from build123d import *

# Parameters (mm, degrees)
F0_R     = 38.2508515855
F1_DEPTH = 17.526
F3_R     = 46.4966196034
F4_DEPTH = 12.7
F5_R     = 5.08
F6_W     = 8.4483027458
F6_H     = 6.8974085152
F8_DEPTH = 9.652
F7_W     = 9.7811389714
F7_H     = 6.7780073732
F9_DEPTH = 10.668


# Not quite as in the source:
# - a fillet or chamfer that OpenCascade refuses, or shapes differently, is made with other operations: its cross-section is extruded or revolved along the edge and cut away or added


with BuildPart() as f1:
    # F0 (on Top) → F1 (new body)
    with BuildSketch(Plane.XY):
        Circle(F0_R)
    extrude(amount=F1_DEPTH)

    # F2: fillet of radius 26.9812507731 on 1 edges, made by hand

    # F2_s1 → F2_t2 (revolve, cut)
    with BuildSketch(Plane.XZ):
        with BuildLine():
            ThreePointArc((38.2508515855, 0), (28.3570882092, 12.7157030349), (12.9805898912, 17.526))
            Line((12.9805898912, 17.526), (38.2508515855, 17.526))
            Line((38.2508515855, 17.526), (38.2508515855, 0))
        make_face()
    revolve(axis=Axis((0, 0, 17.526), (0, 0, 1)), mode=Mode.SUBTRACT)

    # F3 (on face) → F4 (join)
    with BuildSketch(Plane(origin=(0, 0, 0), x_dir=(1, 0, 0), z_dir=(0, 0, -1))):
        Circle(F3_R)
    extrude(amount=F4_DEPTH)

    # F5
    f5_edges = [f1.edges().sort_by_distance(p)[0] for p in [
        (-46.49662, 0, -12.7),
    ]]
    fillet(f5_edges, radius=F5_R)

    # F6 (on face) → F8 (join)
    with BuildSketch(Plane(origin=(0, 0, -12.7), x_dir=(1, 0, 0), z_dir=(0, 0, -1))):
        with Locations((-15.9282591194, 18.548514694)):
            Rectangle(F6_W, F6_H)
    extrude(amount=F8_DEPTH)

    # F7 (on face) → F9 (join)
    with BuildSketch(Plane(origin=(0, 0, -12.7), x_dir=(1, 0, 0), z_dir=(0, 0, -1))):
        with Locations((20.9769504145, -18.5471354052)):
            Rectangle(F7_W, F7_H)
    extrude(amount=F9_DEPTH)


solid = f1.part
For this review, take the finished solid that the model builds, in its own axes (mm). A direction names the side the tool comes from. Round coordinates to 2 decimals unless told otherwise and drop trailing zeros. Write each loop counter-clockwise with the first axis right and the second up, starting at its lowest first coordinate (ties: lowest second). Pieces come first, ordered by that corner, then holes. Notation, with made-up numbers: M -30.75,89.25 L -7.75,89.25 A8 cw -7.75,100.25 Z; hole C 41,-24.75 d9. An arc over 180 degrees is marked long. Write item = value, one per line. Start each with the question number.
(1) For faces 1 (the face through (-16, -15.1, -17)), 2 (the face through (7, 38, 0)), 3 (the face through (-16, -21.997, -17)), 4 (the face through (16.086, 19, -18)), list the 3-axis set-ups (+Z, -Z, +X, -X, +Y, -Y) from which the entire face can be reached by the end or side of a thin tool; tool diameter is ignored.
(2) We need section A-A (z = -1.5). Give the boundary of the cut face in (x, y), then the cut area to 3 significant figures.
(3) For line 1 along Z through (x, y) = (-7, -20.5); line 2 along Z through (x, y) = (11.5, -6); line 3 along X through (y, z) = (-3.5, -7.5), list the stretches that pass through material, from the lowest coordinate up.
(4) The part is to be moulded in two halves that separate along X. For faces 5 (the face through (-11.704, -19, -17)), 6 (the face through (-36.9, 28.29, -3.76)), 7 (the face through (21, 18, -23.368)), say which applies: +X half, -X half, draft (parallel to the pull), parting line (faces both ways), or undercut.
(5) Clearance check with flat-ended pins moving along their axes: pin 1 Ø5.5 at (y, z) = (-19, -19) entering from -X; pin 2 Ø2.5 at (x, z) = (-14, -19) entering from +Y; pin 3 Ø5 at (x, z) = (19, -17) entering from +Y; pin 4 Ø1.5 at (x, z) = (-10.5, -14) entering from +Y. State where each tip first meets the part, or that it passes through.
Results found:
q1.face_1 = -Z, +X, -X, +Y
q1.face_2 = +Z
q1.face_3 = -Z, +X, -X, -Y
q1.face_4 = -Z, -X, +Y, -Y
q2.outline = C 0,0 d92.99
q2.area = 6,790 mm²
q3.line_1 = -12.7 to 16.09
q3.line_2 = -12.7 to 17.53
q3.line_3 = -46.36 to 46.36
q4.face_5 = +X half
q4.face_6 = parting line
q4.face_7 = draft
q5.pin_1 = -20.15
q5.pin_2 = -15.1
q5.pin_3 = 21.94
q5.pin_4 = through
